Geometry: final body of the model. Coordinates: model frame, mm. Face numbers are marked on the shaded views. A direction names the side the tool comes from. Round coordinates to 2 decimals unless told otherwise and drop trailing zeros. Write each loop counter-clockwise with the first axis right and the second up, starting at its lowest first coordinate (ties: lowest second). Pieces come first, ordered by that corner, then holes. Notation, with made-up numbers: (-3.75, -10) -> (33.25, -10) arc R27 ccw to (33.25, 16) -> close; hole circle Ø11 at (36, -22.5). An arc over 180 degrees is marked (long way). Use one line per item in the form item = value. Start each with the question number.
1. Draft query along X for the marked faces 1, 2 and 3. Return one class per face: pulls with the +X half, pulls with the -X half, needs draft (parallel to the pull), parting line crosses it, or undercut.
2. Line query: L1, parallel to Y at x = -20, z = 9.75; L2, parallel to Z at x = -30, y = -10; L3, parallel to Y at x = -9, z = 4.5. Output: solid intervals per line, ascending.
3. Cut plane A-A, the plane y = 0. Return the cut outline in (x, z).
4. Cut plane C-C, the plane y = -12.5. Return the cut outline in (x, z), plus the area to 3 significant figures.
5. Cut plane B-B, the plane z = 1.25. State how many separate pieces and enclosed holes the cut face has, plus the area to 3 significant figures.
6. Cut plane D-D, the plane x = 9. Return the cut outline in (y, z).
7. Pin query (flat end, axial travel): pin 1 Ø3 at (x, y) = (-0.5, 17.5) entering from -Z; pin 2 Ø0.8 at (x, y) = (-22, -10) entering from -Z (3 decimals); pin 3 Ø1.4 at (x, y) = (0, -17.5) entering from -Z. Return the tip coordinate at first contact, or that it passes through.
8. Reachability of the marked faces 4, 5 and 6 from +Z, -Z, +X, -X, +Y, -Y: full face, straight path, thin tool, end or side. Return the list, or none.
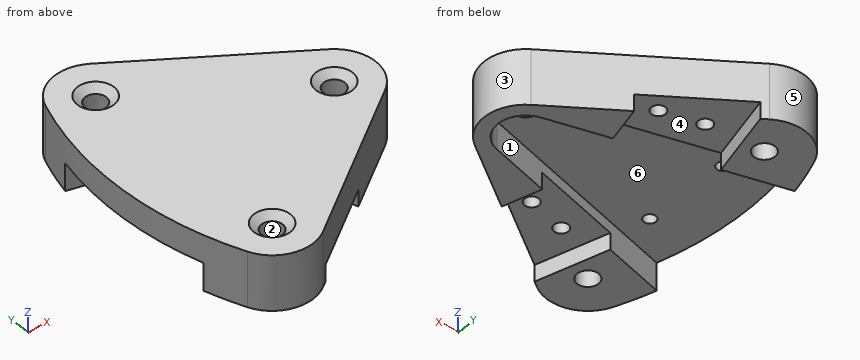
```python
from build123d import *

# Parameters (mm, degrees)
BOSS_EXTRUDE1_DEPTH                               = 12.7
SKETCH2_R                                         = 101.6
SKETCH2_R_2                                       = 76.2
CUT_EXTRUDE1_DEPTH                                = 13.7
FILLET1_R                                         = 9.525
CSK_FOR_8_FLAT_HEAD_MACHINE_SCREW_100_D           = 4.9149
CSK_FOR_8_FLAT_HEAD_MACHINE_SCREW_100_DEPTH       = 12.7
CSK_FOR_8_FLAT_HEAD_MACHINE_SCREW_100_CSINK_D     = 8.4328
CSK_FOR_8_FLAT_HEAD_MACHINE_SCREW_100_CSINK_ANGLE = 100
CUT_EXTRUDE2_DEPTH                                = 6.35
CUT_EXTRUDE3_DEPTH                                = 3.81
SKETCH7_R                                         = 1.397
CUT_EXTRUDE4_DEPTH                                = 3.175
HOLE1_AT_2_COUNT                                  = 2
HOLE1_AT_2_PITCH                                  = 9.3599
HOLE1_AT_3_COUNT                                  = 2
HOLE1_AT_3_PITCH                                  = 38.818175673
HOLE1_AT_4_COUNT                                  = 2
HOLE1_AT_4_PITCH                                  = 40.17317123
F_2_CLEARANCE_HOLE1_D                             = 2.7051
F_2_CLEARANCE_HOLE1_DEPTH                         = 4.7625


with BuildPart() as part:
    # Sketch1 → Boss-Extrude1 (new body)
    with BuildSketch(Plane.XY):
        Polygon((33.299680929, 0), (-33.299680929, 46.0375), (-33.299680929, -46.0375), align=None)
    extrude(amount=BOSS_EXTRUDE1_DEPTH)

    # Sketch2 → Cut-Extrude1 (cut, through all)
    with BuildSketch(Plane.XY.offset(12.7)):
        with Locations((42.900319071, 0)):
            Circle(SKETCH2_R)
        with Locations((42.900319071, 0)):
            Circle(SKETCH2_R_2, mode=Mode.SUBTRACT)
    extrude(amount=-CUT_EXTRUDE1_DEPTH, mode=Mode.SUBTRACT)

    # Fillet1
    fillet1_edges = [part.edges().sort_by_distance(p)[0] for p in [
        (-22.72460624, -38.727369881, 6.35),
        (-22.72460624, 38.727369881, 6.35),
        (33.299680929, 0, 6.35),
    ]]
    fillet(fillet1_edges, radius=FILLET1_R)

    # CSK for #8 Flat Head Machine Screw (100)1
    with Locations(Plane.XY.offset(12.7)):
        with Locations((-19.063658953, -24.617494846), (-19.063658953, 24.617494846), (16.54881886, 0)):
            CounterSinkHole(CSK_FOR_8_FLAT_HEAD_MACHINE_SCREW_100_D / 2, CSK_FOR_8_FLAT_HEAD_MACHINE_SCREW_100_CSINK_D / 2, depth=CSK_FOR_8_FLAT_HEAD_MACHINE_SCREW_100_DEPTH, counter_sink_angle=CSK_FOR_8_FLAT_HEAD_MACHINE_SCREW_100_CSINK_ANGLE)

    # Sketch5 → Cut-Extrude2 (cut)
    with BuildSketch(Plane(origin=(0, 0, 0), x_dir=(-1, 0, 0), z_dir=(0, 0, -1))):
        with BuildLine():
            Line((30.823542048, 19.267389595), (-18.192319797, 6.133628997))
            ThreePointArc((-18.192319797, 6.133628997), (-22.89881886, 0), (-18.192319797, -6.133628997))
            Line((-18.192319797, -6.133628997), (30.823542048, -19.267389595))
            ThreePointArc((30.823542048, -19.267389595), (33.299680929, 0), (30.823542048, 19.267389595))
        make_face()
    extrude(amount=-CUT_EXTRUDE2_DEPTH, mode=Mode.SUBTRACT)

    # Sketch6 → Cut-Extrude3 (cut)
    with BuildSketch(Plane(origin=(0, 0, 0), x_dir=(-1, 0, 0), z_dir=(0, 0, -1))):
        Polygon((16.588726313, -15.453182214), (-4.265612277, -9.86527903), (-8.867414899, -27.039440222), (11.986923691, -32.627343405), align=None)
        Polygon((11.986923691, 32.627343405), (-8.867414899, 27.039440222), (-4.265612277, 9.86527903), (16.588726313, 15.453182214), align=None)
    extrude(amount=-CUT_EXTRUDE3_DEPTH, mode=Mode.SUBTRACT)

    # Sketch7 → Cut-Extrude4 (cut)
    with BuildSketch(Plane(origin=(0, 0, 6.35), x_dir=(-1, 0, 0), z_dir=(0, 0, -1))):
        with Locations((21.479680921, -10.189705806)):
            Circle(SKETCH7_R)
        with Locations((21.479680921, 10.189705806)):
            Circle(SKETCH7_R)
    extrude(amount=-CUT_EXTRUDE4_DEPTH, mode=Mode.SUBTRACT)

    # Sketch9 → Hole1 (revolve, cut)
    with BuildSketch(Plane(origin=(-8.904685942, -20.086585615, 3.81), x_dir=(0, 1, 0), z_dir=(1, 0, 0))):
        Polygon((0, 0), (0, 2.921), (1.4986, 2.921), (1.6383, 0), align=None)
    hole1 = revolve(axis=Axis((-8.904685942, -20.086585615, 113.81), (0, 0, -1)), mode=Mode.SUBTRACT)

    # Hole1 at 2: Hole1 ×2
    with Locations(*[Vector(0.965925826, 0.258819045, 0) * (i * HOLE1_AT_2_PITCH) for i in range(1, HOLE1_AT_2_COUNT)]):
        add(hole1, mode=Mode.SUBTRACT)

    # Hole1 at 3: Hole1 ×2
    with Locations(*[Vector(0.232905565, 0.972499356, 0) * (i * HOLE1_AT_3_PITCH) for i in range(1, HOLE1_AT_3_COUNT)]):
        add(hole1, mode=Mode.SUBTRACT)

    # Hole1 at 4: Hole1 ×2
    with Locations(*[(0, i * HOLE1_AT_4_PITCH, 0) for i in range(1, HOLE1_AT_4_COUNT)]):
        add(hole1, mode=Mode.SUBTRACT)

    # #2 Clearance Hole1
    with Locations(Plane(origin=(0, 0, 3.81), x_dir=(-1, 0, 0), z_dir=(0, 0, -1))):
        with Locations((8.904685942, -20.086585615), (-0.136283199, -17.664065235), (-0.136283199, 17.664065235), (8.904685942, 20.086585615)):
            Hole(F_2_CLEARANCE_HOLE1_D / 2, depth=F_2_CLEARANCE_HOLE1_DEPTH)


solid = part.part
```
Outcome:
q1.face_1 = pulls with the -X half
q1.face_2 = undercut
q1.face_3 = pulls with the +X half
q2.L1 = -34.1 to -26.89, -22.35 to 22.35, 26.89 to 34.1
q2.L2 = 6.35 to 12.7
q2.L3 = -29.24 to -21.69, -18.48 to -13.42, 13.42 to 18.48, 21.69 to 29.24
q3.outline = (-33.3, 6.35) -> (14.09, 6.35) -> (14.09, 11.22) -> (12.33, 12.7) -> (-33.3, 12.7) -> close; (19.01, 6.35) -> (22.9, 6.35) -> (22.9, 0) -> (26.07, 0) -> (26.07, 12.7) -> (20.77, 12.7) -> (19.01, 11.22) -> close
q4.outline = (-32.27, 6.35) -> (-5.57, 6.35) -> (-5.57, 3.81) -> (4.97, 3.81) -> (4.97, 0) -> (15.22, 0) -> (15.22, 12.7) -> (-32.27, 12.7) -> close
q4.area = 393 mm^2
q5.separate_pieces = 3
q5.enclosed_holes = 2
q5.area = 682 mm^2
q6.outline = (-16.8, 0) -> (-8.6, 0) -> (-8.6, 6.35) -> (8.6, 6.35) -> (8.6, 0) -> (16.8, 0) -> (16.8, 12.7) -> (-16.8, 12.7) -> close
q7.pin_1 = 3.81
q7.pin_2 = 9.525
q7.pin_3 = 8.57
q8.face_4 = -Z
q8.face_5 = +Z, -Z, +Y
q8.face_6 = -Z, -X
